For this review, take the finished solid that the model builds, in its own axes (mm). A direction names the side the tool comes from. Round coordinates to 2 decimals unless told otherwise and drop trailing zeros. Order: outer loops, then holes, each group sorted by start corner. A loop starts at its lowest first (then second) coordinate and runs counter-clockwise, first axis right, second up. Notation, with made-up numbers: M 24,20.5 L 46,20.5 A27 cw 46,52.5 Z; hole C 3,-26 d9. An arc over 180 degrees is marked long. Put each result on its own line as item: value.
from build123d import *

# Parameters (mm, degrees)
SKETCH_2_R               = 17.5
EXTRUDE_1_DEPTH          = 10
CUT_EXTRUDE_2_DEPTH      = 10
PATTERN_LINEAR_1_COUNT   = 4
PATTERN_LINEAR_1_PITCH   = 40
SKETCH_6_R               = 1.5
CUT_EXTRUDE_3_DEPTH      = 10
PATTERN_CIRCULAR_1_COUNT = 6


with BuildPart() as part:
    # Эскиз2 → Бобышка-Вытянуть1 (new body)
    with BuildSketch(Plane(origin=(0, 0, 0), x_dir=(0, 0, -1), z_dir=(1, 0, 0))):
        with BuildLine():
            Line((0, 425), (0, 0))
            Line((0, 0), (198, 0))
            Line((198, 0), (71.521752772, 414.791818842))
            ThreePointArc((71.521752772, 414.791818842), (70.382528595, 419.839508404), (70, 425))
            ThreePointArc((70, 425), (35, 460), (0, 425))
        make_face()
        with Locations((35, 425)):
            Circle(SKETCH_2_R, mode=Mode.SUBTRACT)
    extrude(amount=EXTRUDE_1_DEPTH)

    # Эскиз3 → Вырез-Вытянуть2 (cut)
    with BuildSketch(Plane.ZY):
        Polygon((-158, 0), (-158, 7.9), (-159.5, 7.9), (-159.5, 12.1), (-158, 12.1), (-158, 20), (-152.8, 20), (-152.8, 12.1), (-151.3, 12.1), (-151.3, 7.9), (-152.8, 7.9), (-152.8, 0), align=None)
    cut_extrude_2 = extrude(amount=-CUT_EXTRUDE_2_DEPTH, mode=Mode.SUBTRACT)

    # Линейный массив1: Вырез-Вытянуть2 ×4
    with Locations(*[(0, 0, i * PATTERN_LINEAR_1_PITCH) for i in range(1, PATTERN_LINEAR_1_COUNT)]):
        add(cut_extrude_2, mode=Mode.SUBTRACT)

    # Эскиз6 → Вырез-Вытянуть3 (cut)
    with BuildSketch(Plane(origin=(10, 0, 0), x_dir=(0, 0, -1), z_dir=(1, 0, 0))):
        with Locations((8.5, 425)):
            Circle(SKETCH_6_R)
    cut_extrude_3 = extrude(amount=-CUT_EXTRUDE_3_DEPTH, mode=Mode.SUBTRACT)

    # Круговой массив1: Вырез-Вытянуть3 ×6 about axis
    pattern_circular_1_axis = Axis((0, 425, -35), (1, 0, 0))
    for i in range(1, PATTERN_CIRCULAR_1_COUNT):
        add(cut_extrude_3.rotate(pattern_circular_1_axis, i * 360 / PATTERN_CIRCULAR_1_COUNT), mode=Mode.SUBTRACT)


solid = part.part
(1) To check wall thickness, follow L1, parallel to Y at x = 2.75, z = -35; L2, parallel to Y at x = 6.25, z = -48.25; L3, parallel to Y at x = 3, z = -61.5. State the ranges of each line that lie inside material, in increasing order.
A:
L1: y = 20 to 407.5, 442.5 to 460
L2: y = 0 to 400.55, 403.55 to 413.57, 436.43 to 446.45, 449.45 to 457.4
L3: y = 0 to 423.5, 426.5 to 447.86
(2) Insertion check: pin 1 Ø1.2 at (x, z) = (7.5, -79) entering from -Y; pin 2 Ø2 at (x, y) = (7.5, 11) entering from -Z; pin 3 Ø2 at (x, y) = (3.5, 88) entering from -Z; pin 4 Ø4.5 at (x, y) = (7.5, 9) entering from -Z. Each pin has a flat end and moves straight along its axis. Give the tip position at first contact, or say it passes through.
A:
pin 1: stops at y = 0
pin 2: stops at z = -194.95
pin 3: stops at z = -171.47
pin 4: stops at z = -195.94
(3) Draft analysis for pull direction Z (two halves, no side actions). For faces 3 (the face through (5, 0, -55)), 4 (the face through (5, 16, -158)), 5 (the face through (4.93, 204.492, -135.646)), state which applies: released by +Z, released by -Z, zero draft, split by the parting line, or undercut.
A:
face 3: zero draft
face 4: undercut
face 5: released by -Z
(4) Add section A-A on y = 362. Give the boundary of the cut face in (x, z).
A:
outline: M 0,-87.62 L 10,-87.62 L 10,0 L 0,0 Z
(5) Add section B-B on z = -84. Give the boundary of the cut face in (x, y).
A:
outline: M 0,0 L 10,0 L 10,373.87 L 0,373.87 Z
(6) Add section C-C on x = 6.75. State how many separate pieces and enclosed holes the cut face has, then the cut area to 3 significant figures.
A:
separate pieces: 1
enclosed holes: 7
area: 57,100 mm2
(7) For faces 1 (the face through (5, 215, 0)), 2 (the face through (5, 4, -118)), list the 3-axis set-ups (+Z, -Z, +X, -X, +Y, -Y) from which the entire face can be reached by the end or side of a thin tool; tool diameter is ignored.
A:
face 1: +Z, +X, -X, +Y, -Y
face 2: +X, -X, -Y
